Can you work these out from the model? Positions are in its coordinate system, mm. A direction names the side the tool comes from. Coordinates: 2 decimals unless noted, no trailing zeros. Order: outer loops, then holes, each group sorted by start corner. A loop starts at its lowest first (then second) coordinate and runs counter-clockwise, first axis right, second up. Notation, with made-up numbers: (79.25, -13.75) -> (105.25, -13.75) arc R19 ccw to (105.25, -3.75) -> close; hole circle Ø3 at (84.25, 34.25). An arc over 180 degrees is marked (long way). Write item = value, one per line.
```python
from build123d import *

# Parameters (mm, degrees)
SKETCH_1_R               = 6.45
EXTRUDE_1_DEPTH          = 7
SKETCH_2_W               = 29.5
SKETCH_2_H               = 18
EXTRUDE_2_DEPTH          = 3
EXTRUDE_START            = 14.75
SKETCH_3_R               = 1.65
EXTRUDE_3_DEPTH          = 5
EXTRUDE_START_2          = -14.75
SKETCH_3_2_R             = 1.65
EXTRUDE_4_DEPTH          = 5
EXTRUDE_5_DEPTH          = 10
FILLET_1_R               = 5
SKETCH_5_R               = 2.5
CUT_EXTRUDE_1_DEPTH      = 11
CHAMFER_1_SIZE           = 1
CHAMFER_2_SIZE           = 1
CUT_EXTRUDE_2_DEPTH      = 15.75
CUT_EXTRUDE_2_DEPTH_BACK = 15.75
FILLET_2_R               = 1
SKETCH_7_OUTSIDE_W       = 42.194
SKETCH_7_OUTSIDE_H       = 45.694
SKETCH_7_OUTSIDE_R       = 8.66784174
CUT_EXTRUDE_3_DEPTH      = 1
CUT_EXTRUDE_3_DEPTH_BACK = 31


with BuildPart() as part:
    # ｽｹｯﾁ1 → ﾎﾞｽ - 押し出し1 (new body)
    with BuildSketch(Plane.XY):
        Circle(SKETCH_1_R)
    extrude(amount=EXTRUDE_1_DEPTH)

    # ｽｹｯﾁ2 → ﾎﾞｽ - 押し出し2 (add)
    with BuildSketch(Plane.XY.offset(7)):
        Rectangle(SKETCH_2_W, SKETCH_2_H)
    extrude(amount=EXTRUDE_2_DEPTH)

    # ｽｹｯﾁ3 → ﾎﾞｽ - 押し出し3 (add)
    with BuildSketch(Plane(origin=(0, 0, 0), x_dir=(0, 0, -1), z_dir=(1, 0, 0)).offset(EXTRUDE_START)):
        with BuildLine():
            Line((-10, 9), (-23.333333333, 13.714045208))
            ThreePointArc((-23.333333333, 13.714045208), (-29.386897866, 11.398984601), (-28.069570429, 5.053135753))
            Line((-28.069570429, 5.053135753), (-10, -9))
            Line((-10, -9), (-10, 9))
        make_face()
        with Locations((-25, 9)):
            Circle(SKETCH_3_R, mode=Mode.SUBTRACT)
    extrude(amount=-EXTRUDE_3_DEPTH)

    # ｽｹｯﾁ3<2> → ﾎﾞｽ - 押し出し4 (add)
    with BuildSketch(Plane(origin=(0, 0, 0), x_dir=(0, 0, -1), z_dir=(1, 0, 0)).offset(EXTRUDE_START_2)):
        with BuildLine():
            Line((-10, 9), (-23.333333333, 13.714045208))
            ThreePointArc((-23.333333333, 13.714045208), (-29.386897866, 11.398984601), (-28.069570429, 5.053135753))
            Line((-28.069570429, 5.053135753), (-10, -9))
            Line((-10, -9), (-10, 9))
        make_face()
        with Locations((-25, 9)):
            Circle(SKETCH_3_2_R, mode=Mode.SUBTRACT)
    extrude(amount=EXTRUDE_4_DEPTH)

    # ｽｹｯﾁ4 → ﾎﾞｽ - 押し出し5 (add)
    with BuildSketch(Plane.XZ.offset(9)):
        Polygon((-14.75, 7), (14.75, 7), (14.75, 10), (9.75, 10), (-9.75, 10), (-14.75, 10), align=None)
    extrude(amount=EXTRUDE_5_DEPTH)

    # ﾌｨﾚｯﾄ1
    fillet_1_edges = [part.edges().sort_by_distance(p)[0] for p in [
        (-14.75, -19, 8.5),
        (14.75, -19, 8.5),
    ]]
    fillet(fillet_1_edges, radius=FILLET_1_R)

    # ｽｹｯﾁ5 → ｶｯﾄ - 押し出し1 (cut, through all)
    with BuildSketch(Plane.XY.offset(10)):
        with Locations((0, -14)):
            Circle(SKETCH_5_R)
        with Locations((-9.75, -14)):
            Circle(SKETCH_5_R)
        with Locations((9.75, -14)):
            Circle(SKETCH_5_R)
    extrude(amount=-CUT_EXTRUDE_1_DEPTH, mode=Mode.SUBTRACT)

    # 面取り1
    chamfer_1_edges = [part.edges().sort_by_distance(p)[0] for p in [
        (7.25, -14, 7),
        (7.25, -14, 10),
        (-12.25, -14, 7),
        (-12.25, -14, 10),
        (-2.5, -14, 7),
        (-2.5, -14, 10),
    ]]
    chamfer(chamfer_1_edges, length=CHAMFER_1_SIZE)

    # 面取り2
    chamfer_2_edges = [part.edges().sort_by_distance(p)[0] for p in [
        (-14.75, 9, 8.5),
        (0, 9, 7),
        (14.75, 9, 8.5),
        (-14.75, 11.357022604, 16.666666667),
        (-14.75, 11.398984601, 29.386897866),
        (-14.75, -1.973432123, 19.034785215),
        (14.75, 11.357022604, 16.666666667),
        (14.75, 11.398984601, 29.386897866),
        (14.75, -1.973432123, 19.034785215),
    ]]
    chamfer(chamfer_2_edges, length=CHAMFER_2_SIZE)

    # ｽｹｯﾁ6 → ｶｯﾄ - 押し出し2 (cut, two sides)
    with BuildSketch(Plane(origin=(0, 0, 0), x_dir=(0, 0, -1), z_dir=(1, 0, 0))) as cut_extrude_2_sk:
        with BuildLine():
            Line((-5.428941916, -0.825), (-5.905255888, 0))
            Line((-5.905255888, 0), (-5.428941916, 0.825))
            ThreePointArc((-5.428941916, 0.825), (-2.35, 0), (-5.428941916, -0.825))
        make_face()
    extrude(amount=CUT_EXTRUDE_2_DEPTH, mode=Mode.SUBTRACT)
    extrude(cut_extrude_2_sk.sketch, amount=-CUT_EXTRUDE_2_DEPTH_BACK, mode=Mode.SUBTRACT)

    # ﾌｨﾚｯﾄ2
    fillet_2_edges = [part.edges().sort_by_distance(p)[0] for p in [
        (-6.45, 0, 0),
    ]]
    fillet(fillet_2_edges, radius=FILLET_2_R)

    # ｽｹｯﾁ7 outside → ｶｯﾄ - 押し出し3 (cut, two sides)
    with BuildSketch(Plane(origin=(0, 0, 0), x_dir=(-1, 0, 0), z_dir=(0, 0, -1))) as cut_extrude_3_sk:
        with Locations((0, -2.5)):
            Rectangle(SKETCH_7_OUTSIDE_W, SKETCH_7_OUTSIDE_H)
        Circle(SKETCH_7_OUTSIDE_R, mode=Mode.SUBTRACT)
    extrude(amount=CUT_EXTRUDE_3_DEPTH, mode=Mode.SUBTRACT)
    extrude(cut_extrude_3_sk.sketch, amount=-CUT_EXTRUDE_3_DEPTH_BACK, mode=Mode.SUBTRACT)


solid = part.part
```
Item 1: For faces 1 (the flat face through (-0.09, 0.41, 5.67)), 2 (the cylindrical face through (5.96, -2.47, 3.96)), 3 (the flat face through (0, 0, 0)), which set-ups out of +Z, -Z, +X, -X, +Y, -Y let a thin tool reach every point of the face, with its end or its side?
A:
face_1 = +X, -X
face_2 = -Z
face_3 = -Z, +X, -X, +Y, -Y
Item 2: I'm going to push flat-ended pins straight in: P1, Ø1.5, axis at x = 4.5, z = 5.5, coming from the +Y side; P2, Ø6, axis at x = -3.5, z = 6.5, coming from the -Y side; P3, Ø1.5, axis at x = -3.5, y = -5.5, coming from the -Z side. Where does each tip first touch, or does it pass through?
A:
P1 = 5.25
P2 = -8.65
P3 = 0.05
Item 3: I want a section at D-D, the plane y = -7.25. Please give me the cut outline in (x, z).
A:
outline = (-4.75, 7) -> (4.75, 7) -> (4.75, 10) -> (-4.75, 10) -> close
Item 4: I want a section at B-B, the plane z = 9.25. Please give me the cut outline in (x, y).
A:
outline = circle Ø17.34 at (0, 0)
Item 5: I want a section at A-A, the plane x = 0. Please give me the cut outline in (y, z) (3 decimals).
A:
outline = (-8.668, 7) -> (-6.45, 7) -> (-6.45, 1) arc R1 ccw to (-5.45, 0) -> (5.45, 0) arc R1 ccw to (6.45, 1) -> (6.45, 7) -> (8, 7) -> (8.668, 7.668) -> (8.668, 10) -> (-8.668, 10) -> close; hole (-0.825, 5.429) arc R1.65 ccw (long way) to (0.825, 5.429) -> (0, 5.905) -> close
Item 6: If I drill on probe 1 along Y at (x, z) = (3.75, 3.25); probe 2 along Y at (x, z) = (-1.75, 4); probe 3 along Z at (x, y) = (-4.5, -5.75), over which ranges is the centre line in solid material (lowest first)?
A:
probe_1 = -5.25 to -1.47, 1.47 to 5.25
probe_2 = -6.21 to -1.65, 1.65 to 6.21
probe_3 = 7 to 10
Item 7: I want a section at C-C, the plane z = 4.75. Please give me the cut outline in (x, y).
A:
outline = (-6.28, -1.47) arc R6.45 ccw to (6.28, -1.47) -> close; (-6.28, 1.47) -> (6.28, 1.47) arc R6.45 ccw to start
